For this review, take the finished solid that the model builds, in its own axes (mm). A direction names the side the tool comes from. Give positions to 0.01 mm unless a question says otherwise; leave off trailing zeros. Loops run counter-clockwise (first coordinate to the right, second up) from the corner with the lowest first, then second, coordinate; pieces in that order, holes last. Notation, with made-up numbers: (34, 66.5) - (71, 66.5) arc R17 cw to (71, 82.5) - close; hole circle Ø7 at (33.25, 18.25). An arc over 180 degrees is marked (long way). Put each result on its own line as item: value. Start each with the question number.
from build123d import *

# Parameters (mm, degrees)
SKETCH2_W           = 50
SKETCH2_H           = 20
BOSS_EXTRUDE1_DEPTH = 100
SKETCH3_R           = 3.5
CUT_EXTRUDE1_DEPTH  = 114.578166916
SKETCH4_W           = 50
SKETCH4_H           = 20
BOSS_EXTRUDE2_DEPTH = 201
SKETCH5_W           = 50
SKETCH5_H           = 15
BOSS_EXTRUDE3_DEPTH = 60
SKETCH6_R           = 3.5
CUT_EXTRUDE2_DEPTH  = 15
SKETCH7_R           = 6
CUT_EXTRUDE3_DEPTH  = 4
FILLET1_R           = 5
FILLET2_R           = 5
FILLET3_R           = 5
SKETCH15_R          = 6.35
BOSS_EXTRUDE5_DEPTH = 7.9375
MOVE_FACE1_BY       = 1.74
CUT_EXTRUDE9_START  = -7.9375
SKETCH17_R          = 6.35
CUT_EXTRUDE9_DEPTH  = 7.9375
SKETCH16_R          = 25
BOSS_EXTRUDE7_DEPTH = 2.54
SKETCH18_R          = 2.15
CUT_EXTRUDE10_DEPTH = 223.847481476
CUT_EXTRUDE11_START = -2.54
CUT_EXTRUDE11_DEPTH = 2.54
CUT_EXTRUDE12_START = -2.54
SKETCH20_R          = 25
CUT_EXTRUDE12_DEPTH = 2.54
SKETCH21_R          = 5
CUT_EXTRUDE13_DEPTH = 2


with BuildPart() as part:
    # Sketch2 → Boss-Extrude1 (new body)
    with BuildSketch(Plane.XY):
        with Locations((-25, -10)):
            Rectangle(SKETCH2_W, SKETCH2_H)
    boss_extrude1 = extrude(amount=-BOSS_EXTRUDE1_DEPTH)

    # Sketch3 → Cut-Extrude1 (cut, through all)
    with BuildSketch(Plane(origin=(0, 0, 0), x_dir=(1, 0, 0), z_dir=(0, 1, 0))):
        with Locations(Location((-20, 25, 0), (0, 0, 180))):
            Circle(SKETCH3_R)
        with Locations(Location((-35, 20, 0), (0, 0, 180))):
            Circle(SKETCH3_R)
    cut_extrude1 = extrude(amount=-CUT_EXTRUDE1_DEPTH, mode=Mode.SUBTRACT)

    # Sketch4 → Boss-Extrude2 (add)
    with BuildSketch(Plane.XZ.offset(20)):
        with Locations((-25, 10)):
            Rectangle(SKETCH4_W, SKETCH4_H)
    boss_extrude2 = extrude(amount=-BOSS_EXTRUDE2_DEPTH)

    # Sketch5 → Boss-Extrude3 (add)
    with BuildSketch(Plane(origin=(0, 0, 0), x_dir=(-1, 0, 0), z_dir=(0, 0, -1))):
        with Locations((25, 173.5)):
            Rectangle(SKETCH5_W, SKETCH5_H)
    boss_extrude3 = extrude(amount=BOSS_EXTRUDE3_DEPTH)

    # Sketch6 → Cut-Extrude2 (cut)
    with BuildSketch(Plane.XZ.offset(-166)):
        with Locations(Location((-20, -20, 0), (0, 0, 270))):
            Circle(SKETCH6_R)
        with Locations(Location((-20, -40, 0), (0, 0, 270))):
            Circle(SKETCH6_R)
    cut_extrude2 = extrude(amount=-CUT_EXTRUDE2_DEPTH, mode=Mode.SUBTRACT)

    # Sketch7 → Cut-Extrude3 (cut)
    with BuildSketch(Plane(origin=(0, 181, 0), x_dir=(1, 0, 0), z_dir=(0, 1, 0))):
        with Locations(Location((-20, 40, 0), (0, 0, 180))):
            Circle(SKETCH7_R)
        with Locations(Location((-20, 20, 0), (0, 0, 180))):
            Circle(SKETCH7_R)
    cut_extrude3 = extrude(amount=-CUT_EXTRUDE3_DEPTH, mode=Mode.SUBTRACT)

    # Mirror1: Boss-Extrude1, Cut-Extrude1, Boss-Extrude2, Boss-Extrude3, Cut-Extrude2, Cut-Extrude3 across plane
    add(boss_extrude1.mirror(Plane(origin=(0, 0, 0), x_dir=(0, 0, 1), z_dir=(1, 0, 0))))
    add(cut_extrude1.mirror(Plane(origin=(0, 0, 0), x_dir=(0, 0, 1), z_dir=(1, 0, 0))), mode=Mode.SUBTRACT)
    add(boss_extrude2.mirror(Plane(origin=(0, 0, 0), x_dir=(0, 0, 1), z_dir=(1, 0, 0))))
    add(boss_extrude3.mirror(Plane(origin=(0, 0, 0), x_dir=(0, 0, 1), z_dir=(1, 0, 0))))
    add(cut_extrude2.mirror(Plane(origin=(0, 0, 0), x_dir=(0, 0, 1), z_dir=(1, 0, 0))), mode=Mode.SUBTRACT)
    add(cut_extrude3.mirror(Plane(origin=(0, 0, 0), x_dir=(0, 0, 1), z_dir=(1, 0, 0))), mode=Mode.SUBTRACT)

    # Fillet1
    fillet1_edges = [part.edges().sort_by_distance(p)[0] for p in [
        (50, 173.5, -60),
        (-50, -10, -100),
        (0, -20, -100),
        (-50, 173.5, -60),
        (50, -20, -40),
        (50, -10, -100),
        (-50, -20, -40),
    ]]
    fillet(fillet1_edges, radius=FILLET1_R)

    # Fillet2
    fillet2_edges = [part.edges().sort_by_distance(p)[0] for p in [
        (50, 83, 0),
        (-50, 83, 0),
    ]]
    fillet(fillet2_edges, radius=FILLET2_R)

    # Fillet3
    fillet3_edges = [part.edges().sort_by_distance(p)[0] for p in [
        (0, -20, 20),
        (48.535533906, -18.535533906, 20),
        (-48.535533906, -18.535533906, 20),
        (0, 181, -60),
        (48.535533906, 181, -58.535533906),
        (-48.535533906, 181, -58.535533906),
        (-50, 181, -17.5),
        (0, 181, 20),
        (-50, 83, 20),
        (50, 83, 20),
        (50, 181, -17.5),
    ]]
    fillet(fillet3_edges, radius=FILLET3_R)

    # Sketch15 → Boss-Extrude5 (add)
    with BuildSketch(Plane.XY.offset(20)):
        with Locations((0, 80.5)):
            Circle(SKETCH15_R)
    extrude(amount=BOSS_EXTRUDE5_DEPTH)

    # Move Face1: a face moved outward by 1.74
    extrude(part.faces().sort_by_distance((0, 0, -50.320969635))[0], amount=MOVE_FACE1_BY, dir=(0, 1, 0))

    # Sketch17 → Cut-Extrude9 (cut)
    with BuildSketch(Plane.XY.offset(27.9375).offset(CUT_EXTRUDE9_START)):
        with Locations((0, 80.5)):
            Circle(SKETCH17_R)
    extrude(amount=CUT_EXTRUDE9_DEPTH, mode=Mode.SUBTRACT)

    # Sketch16 → Boss-Extrude7 (add)
    with BuildSketch(Plane.XY.offset(20)):
        with Locations((0, 80.5)):
            Circle(SKETCH16_R)
        with BuildLine():
            Line((-20.118015829, 89.945425564), (-1.879029427, 58.354574436))
            ThreePointArc((-1.879029427, 58.354574436), (0, 58.275), (1.879029427, 58.354574436))
            Line((1.879029427, 58.354574436), (20.118015829, 89.945425564))
            ThreePointArc((20.118015829, 89.945425564), (19.247414599, 91.6125), (18.238986403, 93.2))
            Line((18.238986403, 93.2), (-18.238986403, 93.2))
            ThreePointArc((-18.238986403, 93.2), (-19.247414599, 91.6125), (-20.118015829, 89.945425564))
        make_face(mode=Mode.SUBTRACT)
    extrude(amount=BOSS_EXTRUDE7_DEPTH)

    # Sketch18 → Cut-Extrude10 (cut, through all)
    with BuildSketch(Plane.XY.offset(20)):
        with Locations((0, 64.6275)):
            Circle(SKETCH18_R)
        with Locations((-13.748153285, 88.44)):
            Circle(SKETCH18_R)
        with Locations((13.748153285, 88.44)):
            Circle(SKETCH18_R)
    extrude(amount=-CUT_EXTRUDE10_DEPTH, mode=Mode.SUBTRACT)

    # Sketch19 → Cut-Extrude11 (cut)
    with BuildSketch(Plane.XY.offset(20).offset(CUT_EXTRUDE11_START)):
        with BuildLine():
            Line((-20.118015829, 89.945425564), (-1.879029427, 58.354574436))
            ThreePointArc((-1.879029427, 58.354574436), (0, 58.275), (1.879029427, 58.354574436))
            Line((1.879029427, 58.354574436), (20.118015829, 89.945425564))
            ThreePointArc((20.118015829, 89.945425564), (19.247414599, 91.6125), (18.238986403, 93.2))
            Line((18.238986403, 93.2), (-18.238986403, 93.2))
            ThreePointArc((-18.238986403, 93.2), (-19.247414599, 91.6125), (-20.118015829, 89.945425564))
        make_face()
    extrude(amount=CUT_EXTRUDE11_DEPTH, mode=Mode.SUBTRACT)

    # Sketch20 → Cut-Extrude12 (cut)
    with BuildSketch(Plane.XY.offset(22.54).offset(CUT_EXTRUDE12_START)):
        with Locations((0, 80.5)):
            Circle(SKETCH20_R)
    extrude(amount=CUT_EXTRUDE12_DEPTH, mode=Mode.SUBTRACT)

    # Sketch21 → Cut-Extrude13 (cut)
    with BuildSketch(Plane(origin=(0, 0, 0), x_dir=(-1, 0, 0), z_dir=(0, 0, -1))):
        with Locations((-13.748153285, 88.44)):
            Circle(SKETCH21_R)
        with Locations((13.748153285, 88.44)):
            Circle(SKETCH21_R)
        with Locations((0, 64.6275)):
            Circle(SKETCH21_R)
    extrude(amount=-CUT_EXTRUDE13_DEPTH, mode=Mode.SUBTRACT)


solid = part.part
1) Insertion check: P1, Ø2, axis at x = 31.5, y = 7, coming from the -Z side; P2, Ø5, axis at x = 1, y = 64.5, coming from the -Z side; P3, Ø11, axis at x = -20, z = -20, coming from the +Y side. Each pin has a flat end and moves straight along its axis. Give the tip position at first contact, or say it passes through.
2) Take a section at B-B on z = -40. State the section outline as (x, y) points, and give its area (3 significant figures).
3) Mouldability with a two-part tool opening along X and no side actions: class faces 4 (the cylindrical face through (49, -7, -98)), 5 (the cylindrical face through (25.723, 179.028, -18.198)), 6 (the flat face through (1, 83, 0)), 7 (the flat face through (0, 62, 2)) as released by +X, released by -X, zero draft, split by the parting line, or undercut.
4) Wall thickness on probe 1 along X at (y, z) = (172, -20); probe 2 along Y at (x, z) = (-40, -18.5); probe 3 along Z at (x, y) = (-16, 138): over which ranges is each line inside the solid? List them lowest first.
5) Take a section at C-C on z = -7. State the section outline as (x, y) points, and give its area (3 significant figures).
6) Machinability: for faces 1 (the flat face through (-23, 177, -43)), 2 (the cylindrical face through (49, -18, -41)), 3 (the cylindrical face through (-48, 171, -59)), which of the approach directions +Z, -Z, +X, -X, +Y, -Y give a long, thin tool a straight path to every point of the face, cutting with its end or side? Answer none if there is none.
7) Take a section at A-A on x = -35. State the section outline as (y, z) points, and give its area (3 significant figures).
8) Take a section at D-D on z = -86. State the section outline as (x, y) points, and give its area (3 significant figures).
Answers follow:
1. P1: z = 0
1. P2: z = 2
1. P3: y = 177
2. outline: (-50, -15) arc R5 ccw to (-45, -20) - (45, -20) arc R5 ccw to (50, -15) - (50, 1.74) - (-50, 1.74) - close; (-50, 166) - (-23.5, 166) - (-23.5, 177) - (-26, 177) - (-26, 181) - (-45, 181) arc R5 ccw to (-50, 176) - close; (-16.5, 166) - (16.5, 166) - (16.5, 177) - (14, 177) - (14, 181) - (-14, 181) - (-14, 177) - (-16.5, 177) - close; (23.5, 166) - (50, 166) - (50, 176) arc R5 ccw to (45, 181) - (26, 181) - (26, 177) - (23.5, 177) - close
2. area: 3,400 mm2
3. face 4: released by +X
3. face 5: undercut
3. face 6: zero draft
3. face 7: undercut
4. probe 1: -50 to -23.5, -16.5 to 16.5, 23.5 to 50
4. probe 2: -20 to 1.74, 166 to 181
4. probe 3: 0 to 20
5. outline: (-50, -15) arc R5 ccw to (-45, -20) - (45, -20) arc R5 ccw to (50, -15) - (50, 1.74) - (-50, 1.74) - close; (-50, 166) - (50, 166) - (50, 176) arc R5 ccw to (45, 181) - (-45, 181) arc R5 ccw to (-50, 176) - close
5. area: 3,650 mm2
6. face 1: +Y
6. face 2: +Z, -Z, +X, -Y
6. face 3: -Z, -X, +Y
7. outline: (-20, -95) arc R5 ccw to (-15, -100) - (1.74, -100) - (1.74, -23.5) - (-20, -23.5) - close; (-20, -16.5) - (1.74, -16.5) - (1.74, 0) - (166, 0) - (166, -60) - (176, -60) arc R5 ccw to (181, -55) - (181, 15) arc R5 ccw to (176, 20) - (-15, 20) arc R5 ccw to (-20, 15) - close
7. area: 6,920 mm2
8. outline: (-50, -15) arc R5 ccw to (-45, -20) - (45, -20) arc R5 ccw to (50, -15) - (50, 1.74) - (-50, 1.74) - close
8. area: 2,160 mm2
